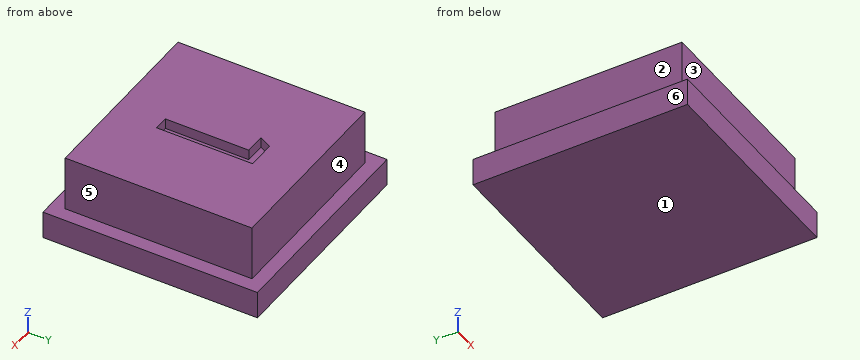
from build123d import *

# Parameters (mm, degrees)
F0_W     = 15.5
F0_H     = 15.5
F0_W_2   = 13.5
F0_H_2   = 13.5
F1_DEPTH = 2
F2_DEPTH = 6
F3_DEPTH = 5.25


with BuildPart() as f1:
    # F0 (on Top) → F1 (new body)
    with BuildSketch(Plane.XY):
        Rectangle(F0_W, F0_H)
        Rectangle(F0_W_2, F0_H_2, mode=Mode.SUBTRACT)
    extrude(amount=F1_DEPTH)

    # F0 (on Top) → F2 (join)
    with BuildSketch(Plane.XY):
        Rectangle(F0_W_2, F0_H_2)
        Polygon((1.24317, -3.46653), (0.205601, -3.46653), (0.205601, 2.567623), (-1.243169, 2.567623), (-0.803279, 3.46653), (1.24317, 3.46653), align=None, mode=Mode.SUBTRACT)
    extrude(amount=F2_DEPTH)

    # F0 (on Top) → F3 (join)
    with BuildSketch(Plane.XY):
        Polygon((0.205601, 2.567623), (0.205601, -3.46653), (1.24317, -3.46653), (1.24317, 3.46653), (-0.803279, 3.46653), (-1.243169, 2.567623), align=None)
    extrude(amount=F3_DEPTH)


solid = f1.part
Model file for the job. Use its own axes, mm. Face numbers are marked on the shaded views. A direction names the side the tool comes from. Coordinates: 2 decimals unless noted, no trailing zeros. Order: outer loops, then holes, each group sorted by start corner. A loop starts at its lowest first (then second) coordinate and runs counter-clockwise, first axis right, second up. Notation, with made-up numbers: M -35.5,46 L -2.5,46 A7 cw -2.5,56 Z; hole C -21,74.25 d10. An arc over 180 degrees is marked long. Return JSON: item names as keys, results as strings.
1. Pull direction X, two halves, no side cores. Call the marked faces 4, 5 and 6: +X half, -X half, draft (parallel to the pull), parting line (faces both ways), or undercut.
Ans:
{"face 4": "draft", "face 5": "+X half", "face 6": "-X half"}
2. Tool access for the marked faces 1, 2 and 3: list every direction of +Z, -Z, +X, -X, +Y, -Y with a clear straight run to the whole face (end or side of a thin tool).
Ans:
{"face 1": "-Z, +X, -X, +Y, -Y", "face 2": "+Z, -X, +Y, -Y", "face 3": "+Z, +X, -X, -Y"}
3. Flat gauge pins, fed straight in: pin 1 (1 mm diameter, centred on x = -4, z = 3, fed in from -Y); pin 2 (2 mm diameter, centred on x = -2.5, z = 3.5, fed in from +Y). Where does each tip first touch, or does it go through?
Ans:
{"pin 1": "y = -6.75", "pin 2": "y = 6.75"}
4. Saw through at B-B (y = 5). Give the cut face in (x, z), and give its area (3 significant figures).
Ans:
{"outline": "M -7.75,0 L 7.75,0 L 7.75,2 L 6.75,2 L 6.75,6 L -6.75,6 L -6.75,2 L -7.75,2 Z", "area": "85.0 mm^2"}
5. Drill centre lines: probe 1 along X at (y, z) = (2.5, 5.5); probe 2 along X at (y, z) = (-4.25, 2.85). Where is each one in solid material? Low to high.
Ans:
{"probe 1": "-6.75 to 0.21, 1.24 to 6.75", "probe 2": "-6.75 to 6.75"}
6. Saw through at D-D (z = 2.2). Give the cut face in (x, y), and give its area (3 significant figures).
Ans:
{"outline": "M -6.75,-6.75 L 6.75,-6.75 L 6.75,6.75 L -6.75,6.75 Z", "area": "182 mm^2"}
7. Saw through at A-A (z = 5.5). Give the cut face in (x, y).
Ans:
{"outline": "M -6.75,-6.75 L 6.75,-6.75 L 6.75,6.75 L -6.75,6.75 Z; hole M -1.24,2.57 L 0.21,2.57 L 0.21,-3.47 L 1.24,-3.47 L 1.24,3.47 L -0.8,3.47 Z"}
